```python
from build123d import *

# Parameters (mm, degrees)
EXTRUDE_1_DEPTH       = 1.2
CUT_EXTRUDE_1_DEPTH   = 1.2
CUT_EXTRUDE_1_2_DEPTH = 1.2
SKETCH_4_R            = 0.6
EXTRUDE_2_DEPTH       = 0.3
SKETCH_5_W            = 29.699213112
SKETCH_5_H            = 7.523800655
EXTRUDE_3_DEPTH       = 0.6


with BuildPart() as part:
    # Эскиз1 → Бобышка-Вытянуть1 (new body)
    with BuildSketch(Plane.XY):
        Polygon((-12.686954911, 6.182258949), (-20.530403447, -0.015033721), (-11.90549662, -6.217213911), (12.642254234, -6.217213911), (20.530403447, 0.015397813), (11.886622261, 6.217213911), (-13.761189247, 6.217213911), align=None)
    extrude(amount=EXTRUDE_1_DEPTH)

    # Эскиз2 → Cut-Extrude 1 (cut)
    with BuildSketch(Plane.XY.offset(1.2)):
        Polygon((-12.686954911, 6.182258949), (-13.761189247, 6.217213911), (-12.642715038, 6.217213911), align=None)
    extrude(amount=-CUT_EXTRUDE_1_DEPTH, mode=Mode.SUBTRACT)

    # Эскиз3 → Cut-Extrude 1 2 (cut)
    with BuildSketch(Plane.XY.offset(1.2)):
        Polygon((11.886622261, 6.217213911), (-12.642715038, 6.217213911), (-20.530403447, -0.015033721), (-11.90549662, -6.217213911), (12.642254234, -6.217213911), (20.530403447, 0.015397813), align=None)
        Polygon((11.757969034, 5.817213911), (-12.503760371, 5.817213911), (-19.866171727, 0), (-11.776608632, -5.817213911), (12.503299567, -5.817213911), (19.865710923, 0), align=None, mode=Mode.SUBTRACT)
    extrude(amount=-CUT_EXTRUDE_1_2_DEPTH, mode=Mode.SUBTRACT)

    # Эскиз4 → Бобышка-Вытянуть2 (add)
    with BuildSketch(Plane.XZ.offset(5.817213911)):
        with Locations(Location((-11.176608632, 0.6, 0), (0, 0, 270))):
            Circle(SKETCH_4_R)
        with Locations(Location((-3.476608632, 0.6, 0), (0, 0, 270))):
            Circle(SKETCH_4_R)
        with Locations(Location((4.223391368, 0.6, 0), (0, 0, 270))):
            Circle(SKETCH_4_R)
        with Locations(Location((11.923391368, 0.6, 0), (0, 0, 270))):
            Circle(SKETCH_4_R)
    extrude(amount=EXTRUDE_2_DEPTH)

    # Эскиз5 → Бобышка-Вытянуть3 (add)
    with BuildSketch(Plane.XZ.offset(6.117213911)):
        with Locations((0.346260417, 0.303007868)):
            Rectangle(SKETCH_5_W, SKETCH_5_H)
    extrude(amount=EXTRUDE_3_DEPTH)


solid = part.part
```
Can you work these out from the model? Positions are in its coordinate system, mm. A direction names the side the tool comes from. Round coordinates to 2 decimals unless told otherwise and drop trailing zeros. Loops run counter-clockwise (first coordinate to the right, second up) from the corner with the lowest first, then second, coordinate; pieces in that order, holes last. Notation, with made-up numbers: M 55,85.5 L 99,85.5 A28 ccw 99,113.5 Z; hole C 56,4.25 d3. An arc over 180 degrees is marked long. Answer as a JSON object with one key per item and string values. Group by question number.
Q1. We'd pull the mould along X, two halves only. Please class faces 4 (the flat face through (0, -5.817, 1)), 5 (the flat face through (0, 0, 1.2)), 6 (the flat face through (-16.13, 2.95, 0.61)): +X half, -X half, draft (parallel to the pull), parting line (faces both ways), or undercut.
Q2. On a 3-axis mill with a long thin cutter (end or side, diameter ignored), from which of +Z, -Z, +X, -X, +Y, -Y can I reach the whole of each face in a straight line? I mean faces 1 (the flat face through (-15.878, -2.868, 0.608)), 2 (the flat face through (0, 0, 0)), 3 (the flat face through (16.13, -2.95, 0.61)). Say none if no direction works.
Q3. Imagine slicing it at A-A, the plane x = 8. Please give me the cut outline in (y, z), then the cut area to 3 significant figures.
Q4. Imagine slicing it at D-D, the plane y = -4. Please give me the cut outline in (x, z).
Q5. Will these pins go through, and if not, where does the flat tip stop? pin 1 (0.7 mm diameter, centred on y = -6.5, z = -0.5, fed in from -X); pin 2 (1.5 mm diameter, centred on x = 13, y = 0, fed in from -Z); pin 3 (4 mm diameter, centred on y = -4, z = 1, fed in from -X).
Q6. Imagine slicing it at B-B, the plane y = -1.5. Please give me the cut outline in (x, z).
Q7. Imagine slicing it at C-C, the plane x = -14. Please give me the cut outline in (y, z) (3 decimals), then the cut area to 3 significant figures.
Q8. Please list where these lines run through material, in increasing order: L1, parallel to Y at x = 3, z = 0.75; L2, parallel to Z at x = -8, y = 3.5; L3, parallel to Y at x = 7, z = 2.5.
Findings:
{
 "1": {"face 4": "undercut", "face 5": "draft", "face 6": "-X half"},
 "2": {"face 1": "+Z, -Z, -X", "face 2": "-Z, +X, -X, +Y", "face 3": "+Z, -Z, +X"},
 "3": {"outline": "M -6.72,-3.46 L -6.12,-3.46 L -6.12,4.06 L -6.72,4.06 Z; M -5.82,0 L 5.82,0 L 5.82,1.2 L -5.82,1.2 Z", "area": "18.5 mm2"},
 "4": {"outline": "M -14.3,0 L 14.8,0 L 14.8,1.2 L -14.3,1.2 Z"},
 "5": {"pin 1": "stops at x = -14.5", "pin 2": "stops at z = 0", "pin 3": "stops at x = -17.08"},
 "6": {"outline": "M -17.78,0 L 17.97,0 L 17.97,1.2 L -17.78,1.2 Z"},
 "7": {"outline": "M -6.717,-3.459 L -6.117,-3.459 L -6.117,4.065 L -6.717,4.065 Z; M -4.218,0 L 4.635,0 L 4.635,1.2 L -4.218,1.2 Z", "area": "15.1 mm2"},
 "8": {"L1": "y = -6.72 to -6.12, -5.82 to 5.82", "L2": "z = 0 to 1.2", "L3": "y = -6.72 to -6.12"}
}
